```python
from build123d import *

# Parameters (mm, degrees)
F0_W     = 31.75
F0_H     = 101.6
F1_DEPTH = 25.4
F2_R     = 10.16
F3_DEPTH = 6.35
F4_R     = 3.175
F5_DEPTH = 3.175
F6_W     = 76.2
F6_H     = 12.7
F7_DEPTH = 31.75


with BuildPart() as f1:
    # F0 (on Right) → F1 (new body)
    with BuildSketch(Plane.YZ):
        with Locations((15.875, 50.8)):
            Rectangle(F0_W, F0_H)
    extrude(amount=-F1_DEPTH)

    # F2 (on face) → F3 (cut)
    with BuildSketch(Plane.YZ):
        with Locations((15.875, 82.55)):
            Circle(F2_R)
    extrude(amount=-F3_DEPTH, mode=Mode.SUBTRACT)

    # F4 (on face) → F5 (cut)
    with BuildSketch(Plane.YZ.offset(-6.35)):
        with Locations((15.875, 82.55)):
            Circle(F4_R)
    extrude(amount=-F5_DEPTH, mode=Mode.SUBTRACT)

    # F6 (on face) → F7 (join)
    with BuildSketch(Plane.XZ):
        with Locations((38.1, 6.35)):
            Rectangle(F6_W, F6_H)
    extrude(amount=-F7_DEPTH)


solid = f1.part
```
Read the model definition and answer for the solid it produces. Units are mm, in the model's axes. A direction names the side the tool comes from. Coordinates: 2 decimals unless noted, no trailing zeros. Order: outer loops, then holes, each group sorted by start corner. A loop starts at its lowest first (then second) coordinate and runs counter-clockwise, first axis right, second up. Notation, with made-up numbers: (16, 13) - (50, 13) arc R23 cw to (50, 40) - close; hole circle Ø1 at (-28, 70.5). An arc over 180 degrees is marked (long way). Answer as a JSON object with one key per item and string values. Group by question number.
Item 1: Flat-ended cylindrical pins translate along their axes: P1, Ø5, axis at x = 1.5, z = 42, coming from the -Y side; P2, Ø12, axis at y = 15.875, z = 82.55, coming from the +X side; P3, Ø16.5, axis at y = 16, z = 86, coming from the +X side; P4, Ø1, axis at x = 24, y = 9, coming from the +Z side. Find the tip coordinate at first contact, or state that the pin passes through.
Item 2: The mould has two halves that part along Y. Classify faces 1 (the face through (0, 16, 58)), 2 (the face through (-9.525, 16, 83)), 3 (the face through (-1, 0, 40)), 4 (the face through (-3.13, 7.81, 76.37)): +Y half, -Y half, draft (parallel to the pull), parting line (faces both ways), or undercut.
Item 3: A tool of negligible diameter and unlimited length cuts with its end or side. For faces 5 (the face through (-25.4, 16, 52)), 6 (the face through (38, 16, 12.7)), 7 (the face through (-6.35, 13, 80)), from which of +Z, -Z, +X, -X, +Y, -Y can it reach the whole face along a straight path? Write none if from no direction.
Item 4: Section A-A (z = 82.55) is taken. Give the vertices of the cut face in (x, y) (3 decimals).
Item 5: Section D-D (z = 16.5) is taken. Give the vertices of the cut face in (x, y).
Item 6: Consider probe 1 along Z at (x, y) = (-3, 16); probe 2 along X at (y, z) = (26, 79.5); probe 3 along Z at (x, y) = (66, 22.5). Determine where each line is inside the solid, lowest interval first. Write a range as from..to.
Item 7: Section C-C (x = 15) is taken. Give the vertices of the cut face in (y, z).
Item 8: Section B-B (y = 17.5) is taken. Give the vertices of the cut face in (x, z) (3 decimals), plus the area to 3 significant figures.
Results are:
{
 "1": {"P1": "stops at y = 0", "P2": "stops at x = -6.35", "P3": "stops at x = 0", "P4": "stops at z = 12.7"},
 "2": {"face 1": "draft", "face 2": "undercut", "face 3": "-Y half", "face 4": "undercut"},
 "3": {"face 5": "+Z, -Z, -X, +Y, -Y", "face 6": "+Z, +X, +Y, -Y", "face 7": "+X"},
 "4": {"outline": "(-25.4, 0) - (0, 0) - (0, 5.715) - (-6.35, 5.715) - (-6.35, 12.7) - (-9.525, 12.7) - (-9.525, 19.05) - (-6.35, 19.05) - (-6.35, 26.035) - (0, 26.035) - (0, 31.75) - (-25.4, 31.75) - close"},
 "5": {"outline": "(-25.4, 0) - (0, 0) - (0, 31.75) - (-25.4, 31.75) - close"},
 "6": {"probe 1": "z = 0..72.39, 92.71..101.6", "probe 2": "x = -25.4..0", "probe 3": "z = 0..12.7"},
 "7": {"outline": "(0, 0) - (31.75, 0) - (31.75, 12.7) - (0, 12.7) - close"},
 "8": {"outline": "(-25.4, 0) - (76.2, 0) - (76.2, 12.7) - (0, 12.7) - (0, 72.521) - (-6.35, 72.521) - (-6.35, 79.822) - (-9.525, 79.822) - (-9.525, 85.278) - (-6.35, 85.278) - (-6.35, 92.579) - (0, 92.579) - (0, 101.6) - (-25.4, 101.6) - close", "area": "3,400 mm^2"}
}
